Input: dimensioned drawing with shaded views. Units: mm. Origin: part minimum x, y, z. A direction names the side the tool comes from. Give positions to 0.01 mm unless a question says otherwise; leave off trailing zeros. Loops run counter-clockwise (first coordinate to the right, second up) from the corner with the lowest first, then second, coordinate; pieces in that order, holes last.
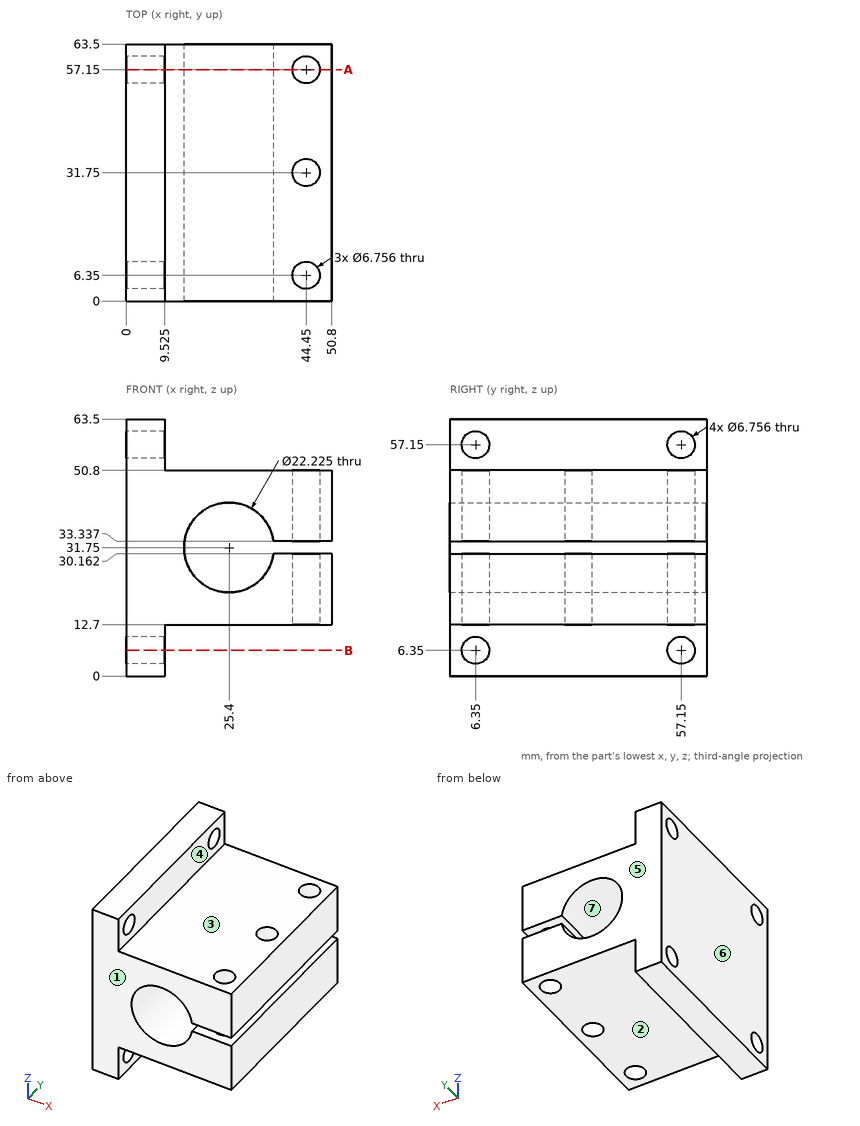
Item 1: Draft query along X for the marked faces 4, 5, 6 and 7. Return one class per face: +X half, -X half, draft (parallel to the pull), parting line (faces both ways), or undercut.
Values follow:
face 4: +X half
face 5: draft
face 6: -X half
face 7: undercut
Item 2: Section query A-A on y = 57.15. Give the number of separate pieces and of enclosed holes in the cut face, plus the area to 3 significant figures.
Values follow:
separate pieces: 5
enclosed holes: 0
area: 1,380 mm2
Item 3: Section query B-B on z = 6.35. Return loops of the section in (x, y) (1 decimal).
Values follow:
outline: (0, 0) - (9.5, 0) - (9.5, 3) - (0, 3) - close; (0, 9.7) - (9.5, 9.7) - (9.5, 53.8) - (0, 53.8) - close; (0, 60.5) - (9.5, 60.5) - (9.5, 63.5) - (0, 63.5) - close
Item 4: Set-up query: the marked faces 1, 2 and 3. Return all of +Z, -Z, +X, -X, +Y, -Y with unobstructed straight access to the full face (end or side cutting, diameter ignored); none if empty.
Values follow:
face 1: +Z, -Z, +X, -X, -Y
face 2: -Z, +X, +Y, -Y
face 3: +Z, +X, +Y, -Y
Item 5: Ray query, probe 1 along Y at (x, z) = (5.5, 6.35); probe 2 along Z at (x, y) = (26, 18); probe 3 along Y at (x, z) = (44.45, 41.75). Return the intervals inside material, ascending.
Values follow:
probe 1: y = 0 to 2.97, 9.73 to 53.77, 60.53 to 63.5
probe 2: z = 12.7 to 20.65, 42.85 to 50.8
probe 3: y = 0 to 2.97, 9.73 to 28.37, 35.13 to 53.77, 60.53 to 63.5
Item 6: Pin query (flat end, axial travel): pin 1 (6 mm diameter, centred on y = 57.15, z = 6.35, fed in from +X); pin 2 (11.5 mm diameter, centred on x = 46, y = 21, fed in from +Z); pin 3 (14 mm diameter, centred on y = 34.5, z = 8.5, fed in from +X); pin 4 (6 mm diameter, centred on x = 17, y = 11, fed in from -Z). Return the tip coordinate at first contact, or that it passes through.
Values follow:
pin 1: passes through
pin 2: stops at z = 50.8
pin 3: stops at x = 50.8
pin 4: stops at z = 12.7
